from build123d import *

# Parameters (mm, degrees)
SKETCH1_R           = 1.322622219
SKETCH1_R_2         = 3.543581518
SKETCH1_W           = 5.363642664
SKETCH1_H           = 3.09972609
BOSS_EXTRUDE1_DEPTH = 3.175


with BuildPart() as part:
    # Sketch1 → Boss-Extrude1 (new body)
    with BuildSketch(Plane(origin=(0, 0, 0), x_dir=(1, 0, 0), z_dir=(0, 1, 0))):
        with BuildLine():
            Line((-30.420224954, 6.394505262), (44.302185909, 6.390032423))
            ThreePointArc((44.302185909, 6.390032423), (50.304735151, 0.387483181), (44.302185909, -5.61506606))
            Line((44.302185909, -5.61506606), (-30.420308604, -5.61506606))
            ThreePointArc((-30.420308604, -5.61506606), (-36.033562007, -7.500021548), (-41.380965097, -4.957001462))
            ThreePointArc((-41.380965097, -4.957001462), (-43.672708861, -3.953506377), (-46.150888165, -3.610404055))
            Line((-46.150888165, -3.610404055), (-48.909665253, -3.610404055))
            ThreePointArc((-48.909665253, -3.610404055), (-52.90984424, 0.389774933), (-48.909665253, 4.38995392))
            Line((-48.909665253, 4.38995392), (-46.150888165, 4.38995392))
            ThreePointArc((-46.150888165, 4.38995392), (-43.564402624, 4.780712621), (-41.208786399, 5.918109658))
            ThreePointArc((-41.208786399, 5.918109658), (-35.908549497, 8.286044856), (-30.420224954, 6.394505262))
        make_face()
        with Locations(Location((44.302185909, 0.387483181, 0), (0, 0, 270))):
            Circle(SKETCH1_R, mode=Mode.SUBTRACT)
        with Locations(Location((0.383109325, 0.385153592, 0), (0, 0, 270))):
            Circle(SKETCH1_R, mode=Mode.SUBTRACT)
        with Locations(Location((-35.559869313, 0.389755399, 0), (0, 0, 270))):
            Circle(SKETCH1_R_2, mode=Mode.SUBTRACT)
        Polygon((34.320012777, 1.885218269), (34.320012777, 1.935143597), (26.334122715, 1.935143597), (26.334122715, 1.885218269), (26.334122715, -1.114852491), (26.334122715, -1.164973144), (34.320012777, -1.164973144), (34.320012777, -1.114852491), align=None, mode=Mode.SUBTRACT)
        with Locations((-9.914943428, 0.385085228)):
            Rectangle(SKETCH1_W, SKETCH1_H, mode=Mode.SUBTRACT)
        with BuildLine():
            Line((-20.582664571, -0.514889121), (-25.573840985, -0.514889121))
            ThreePointArc((-25.573840985, -0.514889121), (-26.473815335, 0.385085229), (-25.573840985, 1.285059578))
            Line((-25.573840985, 1.285059578), (-20.582664571, 1.285059578))
            ThreePointArc((-20.582664571, 1.285059578), (-19.682690221, 0.385085229), (-20.582664571, -0.514889121))
        make_face(mode=Mode.SUBTRACT)
        with BuildLine():
            Line((-49.512218616, 1.385222757), (-45.638080248, 1.385222757))
            ThreePointArc((-45.638080248, 1.385222757), (-44.638040384, 0.385182893), (-45.638080248, -0.614856971))
            Line((-45.638080248, -0.614856971), (-49.512218616, -0.614856971))
            ThreePointArc((-49.512218616, -0.614856971), (-50.51225848, 0.385182893), (-49.512218616, 1.385222757))
        make_face(mode=Mode.SUBTRACT)
    extrude(amount=BOSS_EXTRUDE1_DEPTH)


solid = part.part
Could you check a few things on this model? Use its own coordinates, in mm. A direction names the side the tool comes from. Give positions to 0.01 mm unless a question says otherwise; leave off trailing zeros. Order: outer loops, then holes, each group sorted by start corner. A loop starts at its lowest first (then second) coordinate and runs counter-clockwise, first axis right, second up. Notation, with made-up numbers: (75, 9) -> (110, 9) arc R28 cw to (110, 37) -> close; hole circle Ø6 at (61, -30). An arc over 180 degrees is marked (long way). Return JSON: item names as keys, results as strings.
1. I need wall thicknesses on line 1 (Z direction, x = -35.5, y = 2); line 2 (Z direction, x = -9.5, y = 0.35); line 3 (X direction, y = 0.4, z = 0.75). Which ranges of each line are inside material? Lowest first, please. Write a range as from..to.
Answer list:
{"line 1": "z = -8.29..-3.93, 3.15..7.51", "line 2": "z = -6.39..-1.93, 1.16..5.62", "line 3": "x = -52.74..-38.92, -32.2..-12.6, -7.23..-0.3, 1.06..26.33, 34.32..43.63, 44.98..50.2"}
2. Imagine slicing it at D-D on x = 3. List the corners of the cut face in (y, z) for me (1 decimal), then the cut area to 3 significant figures.
Answer list:
{"outline": "(0, -6.4) -> (3.2, -6.4) -> (3.2, 5.6) -> (0, 5.6) -> close", "area": "38.1 mm2"}
3. Imagine slicing it at C-C on x = -37. List the corners of the cut face in (y, z) for me (1 decimal).
Answer list:
{"outline": "(0, -8.2) -> (3.2, -8.2) -> (3.2, -3.6) -> (0, -3.6) -> close; (0, 2.8) -> (3.2, 2.8) -> (3.2, 7.4) -> (0, 7.4) -> close"}
4. On a 3-axis mill with a long thin cutter (end or side, diameter ignored), from which of +Z, -Z, +X, -X, +Y, -Y can I reach the whole of each face in a straight line? I mean faces 1 (the flat face through (7, 2, 5.615)), 2 (the flat face through (-23, 2, 0.515)), 3 (the flat face through (-1, 3.175, -2)). Say none if no direction works.
Answer list:
{"face 1": "+Z, +X, +Y, -Y", "face 2": "+Y, -Y", "face 3": "+Z, -Z, +X, -X, +Y"}
5. Imagine slicing it at A-A on x = -24. List the corners of the cut face in (y, z) for me (3 decimals).
Answer list:
{"outline": "(0, -6.394) -> (3.175, -6.394) -> (3.175, -1.285) -> (0, -1.285) -> close; (0, 0.515) -> (3.175, 0.515) -> (3.175, 5.615) -> (0, 5.615) -> close"}
6. For pin 1 Ø1.4 at (x, y) = (-48, 2) entering from +Z; pin 2 Ø1 at (x, y) = (29.5, 2) entering from -Z; pin 3 Ø1.6 at (x, y) = (7.5, 2) entering from +Z; pin 4 Ø6.5 at (x, z) = (-35.56, -0.39) entering from +Y, each with a flat end and sliding along its axis, tell me the tip position at first contact or that it passes through.
Answer list:
{"pin 1": "stops at z = 3.61", "pin 2": "stops at z = -6.39", "pin 3": "stops at z = 5.62", "pin 4": "passes through"}
7. Imagine slicing it at B-B on y = 2.15. Give the number of separate pieces and of enclosed holes in the cut face, then the cut area to 3 significant figures.
Answer list:
{"separate pieces": "1", "enclosed holes": "7", "area": "1,090 mm2"}
8. Thinking about a two-plate mould opening in X: for faces 4 (the flat face through (26.334, 2, 0)), 5 (the cylindrical face through (50.303, 1.565, -0.519)), 6 (the flat face through (-48, 2, -4.39)), which applies, pulls with the +X half, pulls with the -X half, needs draft (parallel to the pull), parting line crosses it, or undercut?
Answer list:
{"face 4": "undercut", "face 5": "pulls with the +X half", "face 6": "needs draft"}
